```python
from build123d import *

# Parameters (mm, degrees)
SKETCH2_W           = 18
SKETCH2_H           = 24
SKETCH2_R           = 1
BOSS_EXTRUDE2_DEPTH = 2.5
SKETCH3_W           = 18
SKETCH3_H           = 2.5
BOSS_EXTRUDE3_DEPTH = 21
SKETCH4_W           = 18
SKETCH4_H           = 2.5
BOSS_EXTRUDE4_DEPTH = 17
SKETCH5_W           = 18
SKETCH5_H           = 2.5
BOSS_EXTRUDE5_DEPTH = 42.5


with BuildPart() as part:
    # Sketch2 → Boss-Extrude2 (new body)
    with BuildSketch(Plane(origin=(0, 0, 0), x_dir=(1, 0, 0), z_dir=(0, 1, 0))):
        with Locations((-11, 4)):
            Rectangle(SKETCH2_W, SKETCH2_H)
        with Locations(Location((-17, -6, 0), (0, 0, 270))):
            Circle(SKETCH2_R, mode=Mode.SUBTRACT)
        with Locations(Location((-17, -2, 0), (0, 0, 270))):
            Circle(SKETCH2_R, mode=Mode.SUBTRACT)
        with Locations(Location((-17, 2, 0), (0, 0, 270))):
            Circle(SKETCH2_R, mode=Mode.SUBTRACT)
        with Locations(Location((-17, 6, 0), (0, 0, 270))):
            Circle(SKETCH2_R, mode=Mode.SUBTRACT)
        with Locations(Location((-17, 10, 0), (0, 0, 270))):
            Circle(SKETCH2_R, mode=Mode.SUBTRACT)
        with Locations(Location((-17, 14, 0), (0, 0, 270))):
            Circle(SKETCH2_R, mode=Mode.SUBTRACT)
        with Locations(Location((-13, -4, 0), (0, 0, 270))):
            Circle(SKETCH2_R, mode=Mode.SUBTRACT)
        with Locations(Location((-13, 0, 0), (0, 0, 270))):
            Circle(SKETCH2_R, mode=Mode.SUBTRACT)
        with Locations(Location((-13, 4, 0), (0, 0, 270))):
            Circle(SKETCH2_R, mode=Mode.SUBTRACT)
        with Locations(Location((-13, 8, 0), (0, 0, 270))):
            Circle(SKETCH2_R, mode=Mode.SUBTRACT)
        with Locations(Location((-13, 12, 0), (0, 0, 270))):
            Circle(SKETCH2_R, mode=Mode.SUBTRACT)
        with Locations(Location((-9, -6, 0), (0, 0, 270))):
            Circle(SKETCH2_R, mode=Mode.SUBTRACT)
        with Locations(Location((-9, -2, 0), (0, 0, 270))):
            Circle(SKETCH2_R, mode=Mode.SUBTRACT)
        with Locations(Location((-9, 2, 0), (0, 0, 270))):
            Circle(SKETCH2_R, mode=Mode.SUBTRACT)
        with Locations(Location((-9, 6, 0), (0, 0, 270))):
            Circle(SKETCH2_R, mode=Mode.SUBTRACT)
        with Locations(Location((-9, 10, 0), (0, 0, 270))):
            Circle(SKETCH2_R, mode=Mode.SUBTRACT)
        with Locations(Location((-9, 14, 0), (0, 0, 270))):
            Circle(SKETCH2_R, mode=Mode.SUBTRACT)
        with Locations(Location((-5, -4, 0), (0, 0, 270))):
            Circle(SKETCH2_R, mode=Mode.SUBTRACT)
        with Locations(Location((-5, 0, 0), (0, 0, 270))):
            Circle(SKETCH2_R, mode=Mode.SUBTRACT)
        with Locations(Location((-5, 4, 0), (0, 0, 270))):
            Circle(SKETCH2_R, mode=Mode.SUBTRACT)
        with Locations(Location((-5, 8, 0), (0, 0, 270))):
            Circle(SKETCH2_R, mode=Mode.SUBTRACT)
        with Locations(Location((-5, 12, 0), (0, 0, 270))):
            Circle(SKETCH2_R, mode=Mode.SUBTRACT)
    extrude(amount=BOSS_EXTRUDE2_DEPTH)

    # Sketch3 → Boss-Extrude3 (add)
    with BuildSketch(Plane.XY.offset(8)):
        with Locations((-11, 1.25)):
            Rectangle(SKETCH3_W, SKETCH3_H)
    extrude(amount=BOSS_EXTRUDE3_DEPTH)

    # Sketch4 → Boss-Extrude4 (add)
    with BuildSketch(Plane(origin=(0, 0, 0), x_dir=(-1, 0, 0), z_dir=(0, -1, 0))):
        with Locations((11, -27.75)):
            Rectangle(SKETCH4_W, SKETCH4_H)
    extrude(amount=BOSS_EXTRUDE4_DEPTH)

    # Sketch5 → Boss-Extrude5 (add)
    with BuildSketch(Plane(origin=(0, 0, 26.5), x_dir=(-1, 0, 0), z_dir=(0, 0, -1))):
        with Locations((11, -15.75)):
            Rectangle(SKETCH5_W, SKETCH5_H)
    extrude(amount=BOSS_EXTRUDE5_DEPTH)


solid = part.part
```
Could you check a few things on this model? Use its own coordinates, in mm. A direction names the side the tool comes from. Round coordinates to 2 decimals unless told otherwise and drop trailing zeros. Write each loop counter-clockwise with the first axis right and the second up, starting at its lowest first coordinate (ties: lowest second). Pieces come first, ordered by that corner, then holes.
(1) Suppose I cut it at B-B on z = -6. Write out the boundary of the cut face in (x, y).
Findings below:
outline: (-20, -17) - (-2, -17) - (-2, -14.5) - (-20, -14.5) - close; (-20, 0) - (-18, 0) - (-18, 2.5) - (-20, 2.5) - close; (-16, 0) - (-10, 0) - (-10, 2.5) - (-16, 2.5) - close; (-8, 0) - (-2, 0) - (-2, 2.5) - (-8, 2.5) - close
(2) If I drill on probe 1 along X at (y, z) = (0.5, 6); probe 2 along X at (y, z) = (1.7, 0); probe 3 along Y at (x, z) = (-13.25, -2), over which ranges is the centre line in solid material (lowest first)?
Findings below:
probe 1: x = -20 to -18, -16 to -10, -8 to -2
probe 2: x = -20 to -14, -12 to -6, -4 to -2
probe 3: y = -17 to -14.5, 0 to 2.5
(3) Suppose I cut it at C-C on z = 10. Write out the boundary of the cut face in (x, y), and give its area (3 significant figures).
Findings below:
outline: (-20, -17) - (-2, -17) - (-2, -14.5) - (-20, -14.5) - close; (-20, 0) - (-2, 0) - (-2, 2.5) - (-20, 2.5) - close
area: 90.0 mm2
(4) For pin 1 (3 mm diameter, centred on x = -5, z = 0, fed in from +Y); pin 2 (8 mm diameter, centred on y = -5, z = 0, fed in from -X); pin 3 (1.8 mm diameter, centred on x = -17, z = -14, fed in from +Y), each with a flat end and sliding along its axis, tell me the tip position at first contact or that it passes through.
Findings below:
pin 1: stops at y = 2.5
pin 2: passes through
pin 3: stops at y = -14.5
(5) Which directions (+Z, -Z, +X, -X, +Y, -Y) give clear straight access to the entire face, cutting with the end or side of a thin tool? Please do faces 1 (the face through (-8, 1, -6)), 2 (the face through (-11, 1, -16)).
Findings below:
face 1: +Y
face 2: -Z, +X, -X, +Y, -Y
(6) Suppose I cut it at A-A on x = -5. Write out the boundary of the cut face in (y, z).
Findings below:
outline: (-17, -16) - (-14.5, -16) - (-14.5, 26.5) - (0, 26.5) - (0, 5) - (2.5, 5) - (2.5, 29) - (-17, 29) - close; (0, -16) - (2.5, -16) - (2.5, -13) - (0, -13) - close; (0, -11) - (2.5, -11) - (2.5, -9) - (0, -9) - close; (0, -7) - (2.5, -7) - (2.5, -5) - (0, -5) - close; (0, -3) - (2.5, -3) - (2.5, -1) - (0, -1) - close; (0, 1) - (2.5, 1) - (2.5, 3) - (0, 3) - close
(7) Suppose I cut it at D-D on x = -9. State how many separate pieces and enclosed holes the cut face has, and give its area (3 significant figures).
Findings below:
separate pieces: 7
enclosed holes: 0
area: 231 mm2
(8) Thinking about a two-plate mould opening in X: for faces 3 (the face through (-2, -15, 12)), 4 (the face through (-18, 1, -14)), 5 (the face through (-11, 0, 5)), 6 (the face through (-18, 1, -2)), which applies, +X half, -X half, draft (parallel to the pull), parting line (faces both ways), or undercut?
Findings below:
face 3: +X half
face 4: undercut
face 5: draft
face 6: undercut
